```python
from build123d import *

# Parameters (mm, degrees)
F1_DEPTH = 1.778
F2_D     = 41.91


with BuildPart() as f1:
    # F0 (on Front) → F1 (new body)
    with BuildSketch(Plane.XZ):
        with BuildLine():
            ThreePointArc((35.866425, -70.809534), (50.563695, -80.336742), (48.330608, -62.964617))
            ThreePointArc((48.330608, -62.964617), (42.280856, -67.17678), (35.866425, -70.809534))
        make_face()
        with BuildLine():
            ThreePointArc((30.363654, 73.337843), (37.03637, 70.204686), (43.389643, 66.466003))
            ThreePointArc((43.389643, 66.466003), (44.291812, 83.957815), (30.363654, 73.337843))
        make_face()
        with BuildLine():
            ThreePointArc((-48.330608, 62.964617), (-42.280856, 67.17678), (-35.866425, 70.809534))
            ThreePointArc((-35.866425, 70.809534), (-50.563695, 80.336742), (-48.330608, 62.964617))
        make_face()
        with BuildLine():
            ThreePointArc((78.694262, 10.373226), (79.204633, 5.197769), (79.375, 0))
            ThreePointArc((79.375, 0), (79.345261, -2.17258), (79.256068, -4.343532))
            ThreePointArc((79.256068, -4.343532), (94.855507, 3.621073), (78.694262, 10.373226))
        make_face()
        with BuildLine():
            ThreePointArc((-43.389643, -66.466003), (-44.291812, -83.957815), (-30.363654, -73.337843))
            ThreePointArc((-30.363654, -73.337843), (-37.03637, -70.204686), (-43.389643, -66.466003))
        make_face()
        with BuildLine():
            ThreePointArc((79.256068, -4.343532), (79.345261, -2.17258), (79.375, 0))
            ThreePointArc((79.375, 0), (79.204633, 5.197769), (78.694262, 10.373226))
            ThreePointArc((78.694262, 10.373226), (67.17678, 42.280856), (43.389643, 66.466003))
            ThreePointArc((43.389643, 66.466003), (37.03637, 70.204686), (30.363654, 73.337843))
            ThreePointArc((30.363654, 73.337843), (-3.027905, 79.317226), (-35.866425, 70.809534))
            ThreePointArc((-35.866425, 70.809534), (-42.280856, 67.17678), (-48.330608, 62.964617))
            ThreePointArc((-48.330608, 62.964617), (-70.204686, 37.03637), (-79.256068, 4.343532))
            ThreePointArc((-79.256068, 4.343532), (-79.317226, -3.027905), (-78.694262, -10.373226))
            ThreePointArc((-78.694262, -10.373226), (-67.17678, -42.280856), (-43.389643, -66.466003))
            ThreePointArc((-43.389643, -66.466003), (-37.03637, -70.204686), (-30.363654, -73.337843))
            ThreePointArc((-30.363654, -73.337843), (3.027905, -79.317226), (35.866425, -70.809534))
            ThreePointArc((35.866425, -70.809534), (42.280856, -67.17678), (48.330608, -62.964617))
            ThreePointArc((48.330608, -62.964617), (70.204686, -37.03637), (79.256068, -4.343532))
        make_face()
        with BuildLine():
            ThreePointArc((-78.694262, -10.373226), (-79.317226, -3.027905), (-79.256068, 4.343532))
            ThreePointArc((-79.256068, 4.343532), (-94.855507, -3.621073), (-78.694262, -10.373226))
        make_face()
    extrude(amount=F1_DEPTH)

    # F2 (through all)
    with Locations(Plane(origin=(0, 0, 0), x_dir=(1, 0, 0), z_dir=(0, 1, 0))):
        with Locations((0, 0)):
            Hole(F2_D / 2)


solid = f1.part
```
Verification items for the finished model (mm, model axes). Round coordinates to 2 decimals unless told otherwise and drop trailing zeros. Write each loop counter-clockwise with the first axis right and the second up, starting at its lowest first coordinate (ties: lowest second). Pieces come first, ordered by that corner, then holes.
1. Section check D-D on z = -36. Enter the section's corners in (x, y).
2. Gauge pin test, flat end, axial feed: P1, Ø3, axis at x = -4.5, z = -61, coming from the +Y side. Record the tip position at first contact, or that the pin passes through.
3. Section check B-B on y = -0.45. Enter the section's corners in (x, z) (3 decimals).
4. Draft check along Z on faces 1 (the flat face through (-22, 0, 1)), 2 (the cylindrical face through (-44.56, -0.88, -83.81)). Enter one of: +Z half, -Z half, draft (parallel to the pull), parting line (faces both ways), or undercut.
5. Section check C-C on z = 0. Enter the section's corners in (x, y) (3 decimals).
6. Scan lines: L1, parallel to Z at x = 0, y = -1 (3 decimals); L2, parallel to Z at x = -16.5, y = -1.4; L3, parallel to Z at x = 63, y = -1.15. Record each from-to range of solid material in increasing order.
7. Section check A-A on x = 0. Enter the section's corners in (y, z) (3 decimals), plus the area to 3 significant figures.
Answer:
1. outline: (-70.74, -1.78) - (70.74, -1.78) - (70.74, 0) - (-70.74, 0) - close
2. P1: stops at y = 0
3. outline: (-79.256, 4.344) arc R9.652 ccw (long way) to (-78.694, -10.373) arc R79.375 ccw to (-43.39, -66.466) arc R9.652 ccw (long way) to (-30.364, -73.338) arc R79.375 ccw to (35.866, -70.81) arc R9.652 ccw (long way) to (48.331, -62.965) arc R79.375 ccw to (79.256, -4.344) arc R9.652 ccw (long way) to (78.694, 10.373) arc R79.375 ccw to (43.39, 66.466) arc R9.652 ccw (long way) to (30.364, 73.338) arc R79.375 ccw to (-35.866, 70.81) arc R9.652 ccw (long way) to (-48.331, 62.965) arc R79.375 ccw to start; hole circle Ø41.91 at (0, 0)
4. face 1: draft
4. face 2: undercut
5. outline: (-94.298, -1.778) - (-20.955, -1.778) - (-20.955, 0) - (-94.298, 0) - close; (20.955, -1.778) - (94.298, -1.778) - (94.298, 0) - (20.955, 0) - close
6. L1: z = -79.375 to -20.955, 20.955 to 79.375
6. L2: z = -77.64 to -12.92, 12.92 to 77.64
6. L3: z = -48.28 to 48.28
7. outline: (-1.778, -79.375) - (0, -79.375) - (0, -20.955) - (-1.778, -20.955) - close; (-1.778, 20.955) - (0, 20.955) - (0, 79.375) - (-1.778, 79.375) - close
7. area: 208 mm2
